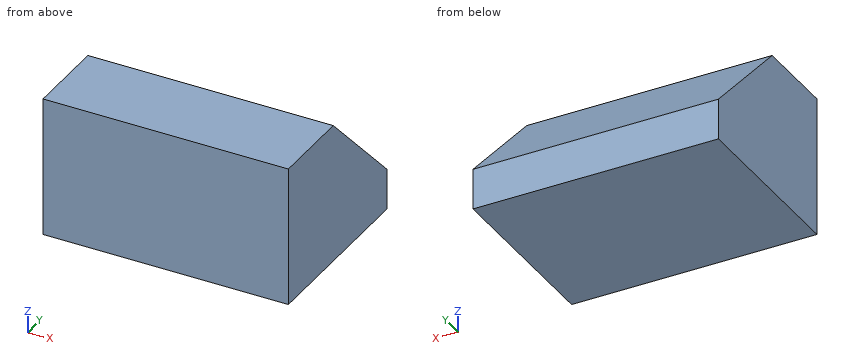
```python
from build123d import *

# Parameters (mm, degrees)
SKIZZE1_W                       = 155.6
SKIZZE1_H                       = 115.2
AUFSATZ_LINEAR_AUSTRAGEN1_DEPTH = 88.8
SCHNITT_LINEAR_AUSTRAGEN1_DEPTH = 189.187566008


with BuildPart() as part:
    # Skizze1 → Aufsatz-Linear austragen1 (new body)
    with BuildSketch(Plane.XY):
        Rectangle(SKIZZE1_W, SKIZZE1_H)
    extrude(amount=AUFSATZ_LINEAR_AUSTRAGEN1_DEPTH)

    # Skizze6 → Schnitt-Linear austragen1 (cut, through all)
    with BuildSketch(Plane.ZY.offset(77.8)):
        Polygon((26.008917831, 57.6), (88.8, -5.191082169), (88.8, 57.6), align=None)
    extrude(amount=-SCHNITT_LINEAR_AUSTRAGEN1_DEPTH, mode=Mode.SUBTRACT)


solid = part.part
```
Build history of the part. All positions in model axes, mm. Give positions to 0.01 mm unless a question says otherwise; leave off trailing zeros. Loops run counter-clockwise (first coordinate to the right, second up) from the corner with the lowest first, then second, coordinate; pieces in that order, holes last.
Item 1: Slice it at B-B, the plane y = 30. List the corners of the cut face in (x, z).
Answers follow:
outline: (-77.8, 0) - (77.8, 0) - (77.8, 53.61) - (-77.8, 53.61) - close
Item 2: Flat gauge pin, fed straight in: pin 1 (6 mm diameter, centred on x = 20.5, y = 9, fed in from +Z). Where does the tip first touch, or does it go through?
Answers follow:
pin 1: stops at z = 77.61
Item 3: Slice it at A-A, the plane x = 16. List the corners of the cut face in (y, z), and give its area (3 significant figures).
Answers follow:
outline: (-57.6, 0) - (57.6, 0) - (57.6, 26.01) - (-5.19, 88.8) - (-57.6, 88.8) - close
area: 8,260 mm2
Item 4: Drill centre lines: line 1 (Z direction, x = 23, y = 38); line 2 (Y direction, x = 57, z = 41.5); line 3 (Y direction, x = -30, z = 36.5). Where is each one in solid material? Low to high.
Answers follow:
line 1: z = 0 to 45.61
line 2: y = -57.6 to 42.11
line 3: y = -57.6 to 47.11
Item 5: Slice it at C-C, the plane z = 73.5. List the corners of the cut face in (x, y), and give its area (3 significant figures).
Answers follow:
outline: (-77.8, -57.6) - (77.8, -57.6) - (77.8, 10.11) - (-77.8, 10.11) - close
area: 10,500 mm2
